Read the model definition and answer for the solid it produces. Units are mm, in the model's axes. A direction names the side the tool comes from. Round coordinates to 2 decimals unless told otherwise and drop trailing zeros. Order: outer loops, then holes, each group sorted by start corner. A loop starts at its lowest first (then second) coordinate and runs counter-clockwise, first axis right, second up. Notation, with made-up numbers: (-33, -16) -> (-22, -16) arc R23 ccw to (-22, 7) -> close; hole circle Ø6 at (-8.5, 24). An arc over 180 degrees is marked (long way). One line per item, written item: value. Start each with the question number.
1. Section C-C (z = -20) is taken. Give the vertices of the cut face in (x, y), then the cut area to 3 significant figures.
2. Section A-A (y = 12) is taken. Give the vertices of the cut face in (x, z), then the cut area to 3 significant figures.
3. Section B-B (x = -14) is taken. Give the vertices of the cut face in (y, z), then the cut area to 3 significant figures.
4. Consider line 1 (Z direction, x = 9, y = -7); line 2 (Z direction, x = 18.5, y = -10); line 3 (Y direction, x = 23, z = 5). Determine where each line is inside the solid, lowest interval first.
5. The mould has two halves that part along Y. Classify faces 1 (the face through (5, -23, -12.7)), 2 (the face through (-23, 0, -12.7)), 3 (the face through (7.795, 21.307, 6.617)): released by +Y, released by -Y, zero draft, split by the parting line, or undercut.
6. Section D-D (y = 18) is taken. Give the vertices of the cut face in (x, z), then the cut area to 3 significant figures.
7. Flat-ended cylindrical pins translate along their axes: pin 1 Ø8 at (y, z) = (-7.5, 6.5) entering from +X; pin 2 Ø1.5 at (x, y) = (-23.5, 1) entering from +Z; pin 3 Ø16.5 at (x, y) = (4, 3.5) entering from +Z. Find the tip coordinate at first contact, or state that the pin passes through.
8. For faces 4 (the face through (22.58, 2.85, 6.62)), 5 (the face through (11.814, 19.454, 6.617)), 6 (the face through (-2.334, -22.64, 6.617)), 7 (the face through (2.18, 22.66, 6.62)), determine the directions among +Z, -Z, +X, -X, +Y, -Y from which every point of the face is accessible in a straight line to the end or side of a thin tool.
from build123d import *

# Parameters (mm, degrees)
F0_R     = 25.4
F1_DEPTH = 25.4
F3_DEPTH = 38.1
F4_R     = 16.51
F5_DEPTH = 2.54


with BuildPart() as f1:
    # F0 (on Top) → F1 (new body, symmetric)
    with BuildSketch(Plane.XY):
        Circle(F0_R)
    extrude(amount=F1_DEPTH, both=True)

    # F2 (on face) → F3 (cut)
    with BuildSketch(Plane.XY.offset(25.4)):
        with BuildLine():
            Line((-4.4029086505, 19.8602374906), (0, 25.4))
            ThreePointArc((0, 25.4), (-5.497566194, 24.7979185808), (-10.7345038482, 23.0202177907))
            Line((-10.7345038482, 23.0202177907), (-4.4029086505, 19.8602374906))
        make_face()
        with BuildLine():
            Line((4.6370208097, 19.7838428525), (11.0425876049, 22.8740302305))
            ThreePointArc((11.0425876049, 22.8740302305), (5.6639046666, 24.7604560525), (0, 25.4))
            Line((0, 25.4), (4.4250969953, 19.83232))
            ThreePointArc((4.4250969953, 19.83232), (4.5311237333, 19.808364842), (4.6370208097, 19.7838428525))
        make_face()
        with BuildLine():
            Line((12.776857167, 15.8004531876), (19.8888569054, 15.7985243297))
            ThreePointArc((19.8888569054, 15.7985243297), (15.865190223, 19.8357187716), (11.0425876049, 22.8740302305))
            Line((11.0425876049, 22.8740302305), (12.6070839942, 15.9362427555))
            ThreePointArc((12.6070839942, 15.9362427555), (12.6921521784, 15.8685750173), (12.776857167, 15.8004531876))
        make_face()
        with BuildLine():
            ThreePointArc((18.2815817765, 8.8705224056), (18.3287717486, 8.7726008794), (18.3754372288, 8.6744283184))
            Line((18.3754372288, 8.6744283184), (24.7793268915, 5.5807668652))
            ThreePointArc((24.7793268915, 5.5807668652), (22.9109646857, 10.9657510992), (19.8888569054, 15.7985243297))
            Line((19.8888569054, 15.7985243297), (18.2815817765, 8.8705224056))
        make_face()
        with BuildLine():
            ThreePointArc((20.319959645, 0.0404972182), (20.3199899113, 0.0202486192), (20.32, 0))
            ThreePointArc((20.32, 0), (20.3198074922, -0.0884504401), (20.3192299724, -0.1768992043))
            Line((20.3192299724, -0.1768992043), (24.7413062764, -5.7469786617))
            ThreePointArc((24.7413062764, -5.7469786617), (25.2347892741, -2.8923019016), (25.4, 0))
            ThreePointArc((25.4, 0), (25.2443548446, 2.8075876616), (24.7793268915, 5.5807668652))
            Line((24.7793268915, 5.5807668652), (20.319959645, 0.0404972182))
        make_face()
        with BuildLine():
            Line((24.7413062764, -5.7469786617), (18.3167939088, -8.7975826738))
            ThreePointArc((18.3167939088, -8.7975826738), (18.2694704717, -8.895439769), (18.2216242397, -8.9930423143))
            Line((18.2216242397, -8.9930423143), (19.78235718, -15.9316773882))
            ThreePointArc((19.78235718, -15.9316773882), (22.8368380896, -11.1192997112), (24.7413062764, -5.7469786617))
        make_face()
        with BuildLine():
            ThreePointArc((10.8887910596, -22.9476410391), (15.7316804593, -19.9417709827), (19.78235718, -15.9316773882))
            Line((19.78235718, -15.9316773882), (12.6705047326, -15.8858650951))
            ThreePointArc((12.6705047326, -15.8858650951), (12.5853443674, -15.9534167862), (12.4998238629, -16.020511958))
            Line((12.4998238629, -16.020511958), (10.8887910596, -22.9476410391))
        make_face()
        with BuildLine():
            ThreePointArc((-0.1705039618, -25.3994277179), (5.497566194, -24.7979185808), (10.8887910596, -22.9476410391))
            Line((10.8887910596, -22.9476410391), (4.5041122558, -19.8145242887))
            ThreePointArc((4.5041122558, -19.8145242887), (4.3980529552, -19.8383348647), (4.291867801, -19.8615777515))
            Line((4.291867801, -19.8615777515), (-0.1705039618, -25.3994277179))
        make_face()
        with BuildLine():
            ThreePointArc((-11.1958865538, -22.799388682), (-5.8299879147, -24.7218777789), (-0.1705039618, -25.3994277179))
            Line((-0.1705039618, -25.3994277179), (-4.5581267877, -19.8021685728))
            ThreePointArc((-4.5581267877, -19.8021685728), (-4.6639903317, -19.7775022231), (-4.7697204121, -19.752269925))
            Line((-4.7697204121, -19.752269925), (-11.1958865538, -22.799388682))
        make_face()
        with BuildLine():
            ThreePointArc((-19.9944604075, -15.6646593648), (-15.9979850762, -19.7287727318), (-11.1958865538, -22.799388682))
            Line((-11.1958865538, -22.799388682), (-12.7137760303, -15.8512554409))
            ThreePointArc((-12.7137760303, -15.8512554409), (-12.798388061, -15.7830181854), (-12.882633856, -15.7143292868))
            Line((-12.882633856, -15.7143292868), (-19.9944604075, -15.6646593648))
        make_face()
        with BuildLine():
            ThreePointArc((-24.816230911, -5.4143035905), (-22.9840588775, -10.8117083532), (-19.9944604075, -15.6646593648))
            Line((-19.9944604075, -15.6646593648), (-18.3407155164, -8.7476027772))
            ThreePointArc((-18.3407155164, -8.7476027772), (-18.387247102, -8.6493666825), (-18.4332525225, -8.5508830796))
            Line((-18.4332525225, -8.5508830796), (-24.816230911, -5.4143035905))
        make_face()
        with BuildLine():
            Line((-20.3175846832, 0.313293219), (-24.7021707789, 5.9129314903))
            ThreePointArc((-24.7021707789, 5.9129314903), (-25.3987123714, 0.2557535417), (-24.816230911, -5.4143035905))
            Line((-24.816230911, -5.4143035905), (-20.3197736682, 0.0959065927))
            ThreePointArc((-20.3197736682, 0.0959065927), (-20.3189698971, 0.2046028333), (-20.3175846832, 0.313293219))
        make_face()
        with BuildLine():
            Line((-18.1608456078, 9.1151569822), (-19.6749660304, 16.0641125401))
            ThreePointArc((-19.6749660304, 16.0641125401), (-22.7616824296, 11.27234727), (-24.7021707789, 5.9129314903))
            Line((-24.7021707789, 5.9129314903), (-18.2573252052, 8.9203405963))
            ThreePointArc((-18.2573252052, 8.9203405963), (-18.2093459437, 9.017877816), (-18.1608456078, 9.1151569822))
        make_face()
        with BuildLine():
            Line((-12.3920004699, 16.1040592508), (-10.7345038482, 23.0202177907))
            ThreePointArc((-10.7345038482, 23.0202177907), (-15.5974618012, 20.0469245861), (-19.6749660304, 16.0641125401))
            Line((-19.6749660304, 16.0641125401), (-12.5635813453, 15.9705611604))
            ThreePointArc((-12.5635813453, 15.9705611604), (-12.4779694409, 16.0375396689), (-12.3920004699, 16.1040592508))
        make_face()
    extrude(amount=-F3_DEPTH, mode=Mode.SUBTRACT)

    # F4 (on face) → F5 (cut)
    with BuildSketch(Plane.XY.offset(25.4)):
        Circle(F4_R)
    extrude(amount=-F5_DEPTH, mode=Mode.SUBTRACT)


solid = f1.part
Answer:
1. outline: circle Ø50.8 at (0, 0)
1. area: 2,030 mm^2
2. outline: (-22.39, -25.4) -> (22.39, -25.4) -> (22.39, -12.7) -> (19.01, -12.7) -> (19.01, 25.4) -> (11.34, 25.4) -> (11.34, 22.86) -> (-11.34, 22.86) -> (-11.34, 25.4) -> (-18.79, 25.4) -> (-18.79, -12.7) -> (-22.39, -12.7) -> close
2. area: 1,950 mm^2
3. outline: (-21.19, -25.4) -> (21.19, -25.4) -> (21.19, -12.7) -> (15.99, -12.7) -> (15.99, 25.4) -> (8.75, 25.4) -> (8.75, 22.86) -> (-8.75, 22.86) -> (-8.75, 25.4) -> (-15.71, 25.4) -> (-15.71, -12.7) -> (-21.19, -12.7) -> close
3. area: 1,700 mm^2
4. line 1: -25.4 to 22.86
4. line 2: -25.4 to -12.7
4. line 3: -6.57 to -3.55, 3.37 to 6.44
5. face 1: zero draft
5. face 2: undercut
5. face 3: released by +Y
6. outline: (-17.92, -25.4) -> (17.92, -25.4) -> (17.92, -12.7) -> (12.14, -12.7) -> (12.14, 25.4) -> (-11.94, 25.4) -> (-11.94, -12.7) -> (-17.92, -12.7) -> close
6. area: 1,370 mm^2
7. pin 1: x = 24.74
7. pin 2: z = -12.7
7. pin 3: z = 22.86
8. face 4: +Z, +X
8. face 5: +Z, +X, +Y
8. face 6: +Z, -Y
8. face 7: +Z, +Y
